Part model, mm, in its own coordinate system. A direction names the side the tool comes from. Round coordinates to 2 decimals unless told otherwise and drop trailing zeros. Order: outer loops, then holes, each group sorted by start corner. A loop starts at its lowest first (then second) coordinate and runs counter-clockwise, first axis right, second up. Notation, with made-up numbers: (-8.75, 64) -> (41.25, 64) arc R28 ccw to (41.25, 88) -> close; hole circle Ø8 at (-20.75, -22). An arc over 180 degrees is marked (long way). Use CSV: the item, a comma, the result in double quotes.
```python
from build123d import *

# Parameters (mm, degrees)
F0_W     = 74
F0_H     = 42.9
F0_R     = 1.6
F1_DEPTH = 1.6
F2_W     = 60.26
F2_H     = 42.72
F3_DEPTH = 4.7
F4_W     = 48.96
F4_H     = 38
F5_DEPTH = 0.1
F6_W     = 15
F6_H     = 15
F7_DEPTH = 2
F6_W_2   = 8
F8_DEPTH = 6
F9_R     = 3


with BuildPart() as f1:
    # F0 (on Top) → F1 (new body)
    with BuildSketch(Plane.XY):
        Rectangle(F0_W, F0_H)
        with Locations((-34, -18.36)):
            Circle(F0_R, mode=Mode.SUBTRACT)
        with Locations((34, -18.36)):
            Circle(F0_R, mode=Mode.SUBTRACT)
        with Locations((-34, 18.36)):
            Circle(F0_R, mode=Mode.SUBTRACT)
        with Locations((34, 18.36)):
            Circle(F0_R, mode=Mode.SUBTRACT)
    extrude(amount=F1_DEPTH)

    # F2 (on face) → F3 (join)
    with BuildSketch(Plane.XY.offset(1.6)):
        with Locations((0, -0.01)):
            Rectangle(F2_W, F2_H)
    extrude(amount=F3_DEPTH)

    # F4 (on face) → F5 (cut)
    with BuildSketch(Plane.XY.offset(6.3)):
        with Locations((0, 0.35)):
            Rectangle(F4_W, F4_H)
    extrude(amount=-F5_DEPTH, mode=Mode.SUBTRACT)

    # F6 (on face) → F7 (join)
    with BuildSketch(Plane(origin=(0, 0, 0), x_dir=(1, 0, 0), z_dir=(0, 0, -1))):
        with Locations((-15.5, 13.95)):
            Rectangle(F6_W, F6_H)
    extrude(amount=F7_DEPTH)

    # F6 (on face) → F8 (join)
    with BuildSketch(Plane(origin=(0, 0, 0), x_dir=(1, 0, 0), z_dir=(0, 0, -1))):
        with Locations((-33, 0)):
            Rectangle(F6_W_2, F6_H)
    extrude(amount=F8_DEPTH)

    # F9
    f9_edges = [f1.edges().sort_by_distance(p)[0] for p in [
        (37, 21.45, 0.8),
        (37, -21.45, 0.8),
        (-37, -21.45, 0.8),
        (-37, 21.45, 0.8),
    ]]
    fillet(f9_edges, radius=F9_R)


solid = f1.part
```
(1) Cut at D-D, the plane x = 27. Give the cut face in (y, z).
Reply:
outline,"(-21.45, 0) -> (21.45, 0) -> (21.45, 1.6) -> (21.35, 1.6) -> (21.35, 6.3) -> (-21.37, 6.3) -> (-21.37, 1.6) -> (-21.45, 1.6) -> close"
(2) Cut at B-B, the plane x = -21. Give the cut face in (y, z), then the cut area to 3 significant figures.
Reply:
outline,"(-21.45, -2) -> (-6.45, -2) -> (-6.45, 0) -> (21.45, 0) -> (21.45, 1.6) -> (21.35, 1.6) -> (21.35, 6.3) -> (19.35, 6.3) -> (19.35, 6.2) -> (-18.65, 6.2) -> (-18.65, 6.3) -> (-21.37, 6.3) -> (-21.37, 1.6) -> (-21.45, 1.6) -> close"
area,"296 mm2"
(3) Probe probe 1 along Y at (x, z) = (34, 1.1); probe 2 along Z at (x, y) = (-14, -10); probe 3 along Z at (x, y) = (-4.5, -1.5). List the from-to ranges inside material, lowest first. Write a range as [from, to].
Reply:
probe 1,"[-21.45, -19.96], [-16.76, 16.76], [19.96, 21.45]"
probe 2,"[-2, 6.2]"
probe 3,"[0, 6.2]"
(4) Which spindle directions (+Z, -Z, +X, -X, +Y, -Y) get a long thin tool onto all of the face, cutting with end or side? Do faces 4 (the face through (-33, 7.5, -3)), 5 (the face through (-16, -6.45, -1)), 6 (the face through (-8, -14, -1)), 7 (the face through (0, -21.37, 4)), 8 (the face through (30.13, 0, 4)). Say none if no direction does.
Reply:
face 4,"-Z, +X, -X, +Y"
face 5,"-Z, +X, +Y"
face 6,"-Z, +X, +Y, -Y"
face 7,"+Z, +X, -X, -Y"
face 8,"+Z, +X, +Y, -Y"
(5) Cut at A-A, the plane y = -4. Give the cut face in (x, z), then the cut area to 3 significant figures.
Reply:
outline,"(-37, -6) -> (-29, -6) -> (-29, 0) -> (37, 0) -> (37, 1.6) -> (30.13, 1.6) -> (30.13, 6.3) -> (24.48, 6.3) -> (24.48, 6.2) -> (-24.48, 6.2) -> (-24.48, 6.3) -> (-30.13, 6.3) -> (-30.13, 1.6) -> (-37, 1.6) -> close"
area,"445 mm2"
(6) Cut at C-C, the plane y = -12.5. Give the cut face in (x, z), then the cut area to 3 significant figures.
Reply:
outline,"(-37, 0) -> (-23, 0) -> (-23, -2) -> (-8, -2) -> (-8, 0) -> (37, 0) -> (37, 1.6) -> (30.13, 1.6) -> (30.13, 6.3) -> (24.48, 6.3) -> (24.48, 6.2) -> (-24.48, 6.2) -> (-24.48, 6.3) -> (-30.13, 6.3) -> (-30.13, 1.6) -> (-37, 1.6) -> close"
area,"427 mm2"
(7) Pull direction Y, two halves, no side cores. Call faces 1 (the face through (-33, -7.5, -3)), 2 (the face through (0, 21.35, 4)), 3 (the face through (-35.6, -18.3, 0.8)): released by +Y, released by -Y, zero draft, split by the parting line, or undercut.
Reply:
face 1,"released by -Y"
face 2,"released by +Y"
face 3,"undercut"
(8) Drop flat-ended pins along their axis: P1, Ø2, axis at x = 12.5, y = -7.5, coming from the -Z side; P2, Ø2.5, axis at x = -10, z = 4, coming from the -Y side; P3, Ø1, axis at y = -5, z = 3, coming from the -X side; P4, Ø3, axis at x = 34, y = 18.36, coming from the -Z side. Give the stop position or say it passes through.
Reply:
P1,"z = 0"
P2,"y = -21.37"
P3,"x = -30.13"
P4,"through"
